```python
from build123d import *

# Parameters (mm, degrees)
BOSS_EXTRUDE1_DEPTH = 5
FILLET1_R           = 10
CUT_EXTRUDE1_DEPTH  = 0.5


with BuildPart() as part:
    # Sketch1 → Boss-Extrude1 (new body)
    with BuildSketch(Plane.XY):
        with BuildLine():
            ThreePointArc((32.82300848, 7.156370874), (9.466254973, 44.595523799), (-34.426436475, 49.140822863))
            ThreePointArc((-34.426436475, 49.140822863), (-38.572797774, 45.958016405), (-42.426406871, 42.426406871))
            ThreePointArc((-42.426406871, 42.426406871), (-26.29235792, 40.654943242), (-22.609103215, 24.847373735))
            ThreePointArc((-22.609103215, 24.847373735), (-43.353983992, -14.099744614), (-25.343982725, -54.38457998))
            ThreePointArc((-25.343982725, -54.38457998), (-20.514410827, -56.38403097), (-15.529142706, -57.955549577))
            ThreePointArc((-15.529142706, -57.955549577), (-22.062034677, -43.097321505), (-10.213905264, -32.003744609))
            ThreePointArc((-10.213905264, -32.003744609), (33.887729018, -30.495779185), (59.7704192, 5.243757117))
            ThreePointArc((59.7704192, 5.243757117), (59.087208601, 10.426014565), (57.955549577, 15.529142706))
            ThreePointArc((57.955549577, 15.529142706), (48.354392597, 2.442378263), (32.82300848, 7.156370874))
        make_face()
        with BuildLine():
            Line((-3.983032008, 15.390433913), (-14.46497239, 6.595041605))
            ThreePointArc((-14.46497239, 6.595041605), (-14.855921916, 6.412738847), (-15.285645517, 6.45033479))
            ThreePointArc((-15.285645517, 6.45033479), (-16.353739487, 5.952274392), (-15.855679089, 4.884180422))
            ThreePointArc((-15.855679089, 4.884180422), (-15.502325506, 4.63675958), (-15.320022748, 4.245810053))
            Line((-15.320022748, 4.245810053), (-12.943959764, -9.229512752))
            ThreePointArc((-12.943959764, -9.229512752), (-12.981555707, -9.659236353), (-13.22897655, -10.012589936))
            ThreePointArc((-13.22897655, -10.012589936), (-13.331690578, -11.186616647), (-12.157663867, -11.289330674))
            ThreePointArc((-12.157663867, -11.289330674), (-11.76671434, -11.107027916), (-11.336990739, -11.14462386))
            Line((-11.336990739, -11.14462386), (1.521012626, -15.824554357))
            ThreePointArc((1.521012626, -15.824554357), (1.874366209, -16.071975199), (2.056668967, -16.462924726))
            ThreePointArc((2.056668967, -16.462924726), (3.02204891, -17.138891039), (3.698015222, -16.173511097))
            ThreePointArc((3.698015222, -16.173511097), (3.735611166, -15.743787496), (3.983032008, -15.390433913))
            Line((3.983032008, -15.390433913), (14.46497239, -6.595041605))
            ThreePointArc((14.46497239, -6.595041605), (14.855921916, -6.412738847), (15.285645517, -6.45033479))
            ThreePointArc((15.285645517, -6.45033479), (16.353739487, -5.952274392), (15.855679089, -4.884180422))
            ThreePointArc((15.855679089, -4.884180422), (15.502325506, -4.63675958), (15.320022748, -4.245810053))
            Line((15.320022748, -4.245810053), (12.943959764, 9.229512752))
            ThreePointArc((12.943959764, 9.229512752), (12.981555707, 9.659236353), (13.22897655, 10.012589936))
            ThreePointArc((13.22897655, 10.012589936), (13.331690578, 11.186616647), (12.157663867, 11.289330674))
            ThreePointArc((12.157663867, 11.289330674), (11.76671434, 11.107027916), (11.336990739, 11.14462386))
            Line((11.336990739, 11.14462386), (-1.521012626, 15.824554357))
            ThreePointArc((-1.521012626, 15.824554357), (-1.874366209, 16.071975199), (-2.056668967, 16.462924726))
            ThreePointArc((-2.056668967, 16.462924726), (-3.02204891, 17.138891039), (-3.698015222, 16.173511097))
            ThreePointArc((-3.698015222, 16.173511097), (-3.735611166, 15.743787496), (-3.983032008, 15.390433913))
        make_face(mode=Mode.SUBTRACT)
    extrude(amount=BOSS_EXTRUDE1_DEPTH)

    # Fillet1
    fillet1_edges = [part.edges().sort_by_distance(p)[0] for p in [
        (32.82300848, 7.156370874, 2.5),
        (-10.213905264, -32.003744609, 2.5),
        (-22.609103215, 24.847373735, 2.5),
    ]]
    fillet(fillet1_edges, radius=FILLET1_R)

    # Sketch2 → Cut-Extrude1 (cut)
    with BuildSketch(Plane.XY.offset(5)):
        Polygon((2.689022882, -16.689899207), (3.181426759, -16.603075118), (4.917908536, -26.451152648), (4.425504659, -26.537976737), align=None)
        Polygon((15.798388141, -6.016187476), (15.969398213, -5.546341165), (25.36632442, -8.966542599), (25.195314349, -9.436388909), align=None)
    extrude(amount=-CUT_EXTRUDE1_DEPTH, mode=Mode.SUBTRACT)


solid = part.part
```
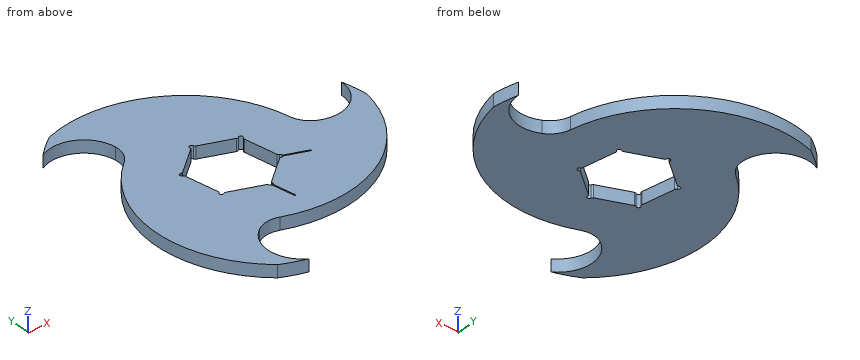
The model under review builds one solid part; all positions refer to its coordinate system, in mm. Coordinates: 2 decimals unless noted, no trailing zeros. Order: outer loops, then holes, each group sorted by start corner. A loop starts at its lowest first (then second) coordinate and runs counter-clockwise, first axis right, second up. Notation, with made-up numbers: M 41,74 L 48,74 A23 cw 48,109 Z; hole C -3.75,89 d2. An arc over 180 degrees is marked long. One line per question, with ' | ' between items.
(1) Add section C-C, the plane x = 42.5. Write out the cut boundary in (y, z).
Geometry results:
outline: M -24.7,0 L 1.79,0 L 1.79,5 L -24.7,5 Z
(2) Add section B-B, the plane y = 36. Write out the cut boundary in (x, z).
Geometry results:
outline: M -22.85,0 L 19.83,0 L 19.83,5 L -22.85,5 Z
(3) Add section A-A, the plane x = -28. Write out the cut boundary in (y, z), then the cut area to 3 significant figures.
Geometry results:
outline: M -52,0 L 20.34,0 L 20.34,5 L -52,5 Z; M 41.95,0 L 51.02,0 L 51.02,5 L 41.95,5 Z | area: 407 mm²
(4) For probe 1 along X at (y, z) = (-10, 0.35); probe 2 along Y at (x, z) = (-8.5, 4.75); probe 3 along Y at (x, z) = (-11.5, 1.4), list the stretches that pass through material, from the lowest coordinate up. Write a range as from..to.
Geometry results:
probe 1: x = -43.04..-13.21, 10.41..54.49 | probe 2: y = -32.86..-12.18, 11.6..51.47 | probe 3: y = -32.66..-11.1, 9.08..51.9
(5) Insertion check: pin 1 (4 mm diameter, centred on x = 19, y = -7, fed in from +Z); pin 2 (1.5 mm diameter, centred on x = 7, z = 2.5, fed in from +Y); pin 3 (1.5 mm diameter, centred on x = 49, z = 3, fed in from +Y). Each pin has a flat end and moves straight along its axis. Give the tip position at first contact, or say it passes through.
Geometry results:
pin 1: stops at z = 5 | pin 2: stops at y = 46.44 | pin 3: stops at y = 2.99
